from build123d import *

# Parameters (mm, degrees)
BOSS_EXTRUDE1_DEPTH = 1.5


with BuildPart() as part:
    # Sketch1 → Boss-Extrude1 (new body, symmetric)
    with BuildSketch(Plane(origin=(0, 0, 0), x_dir=(1, 0, 0), z_dir=(0, 1, 0))):
        with BuildLine():
            Line((-94.5, 0), (-88.5, 0))
            Line((-88.5, 0), (-88.5, 5))
            Line((-88.5, 5), (-84, 5))
            ThreePointArc((-84, 5), (0, 89), (84, 5))
            Line((84, 5), (88.5, 5))
            Line((88.5, 5), (88.5, 0))
            Line((88.5, 0), (94.5, 0))
            Line((94.5, 0), (94.5, 5))
            Line((94.5, 5), (99, 5))
            ThreePointArc((99, 5), (0, 104), (-99, 5))
            Line((-99, 5), (-94.5, 5))
            Line((-94.5, 5), (-94.5, 0))
        make_face()
    extrude(amount=BOSS_EXTRUDE1_DEPTH, both=True)


solid = part.part
Could you check a few things on this model? Use its own coordinates, in mm. Round coordinates to 2 decimals unless told otherwise and drop trailing zeros. Order: outer loops, then holes, each group sorted by start corner. A loop starts at its lowest first (then second) coordinate and runs counter-clockwise, first axis right, second up.
Q1. Imagine slicing it at D-D, the plane x = -59. List the corners of the cut face in (y, z) for me.
Geometry says:
outline: (-1.5, -84.5) - (1.5, -84.5) - (1.5, -64.79) - (-1.5, -64.79) - close
Q2. Please list where these lines run through material, in increasing order: probe 1 along X at (y, z) = (1.1, -21); probe 2 along X at (y, z) = (-0.2, -36); probe 3 along Z at (x, y) = (72, 0.8).
Geometry says:
probe 1: x = -97.7 to -82.46, 82.46 to 97.7
probe 2: x = -94.02 to -78.07, 78.07 to 94.02
probe 3: z = -72.95 to -48.27
Q3. Imagine slicing it at B-B, the plane y = -0.9. List the corners of the cut face in (x, z) for me.
Geometry says:
outline: (-99, -5) arc R99 ccw to (99, -5) - (94.5, -5) - (94.5, 0) - (88.5, 0) - (88.5, -5) - (84, -5) arc R84 cw to (-84, -5) - (-88.5, -5) - (-88.5, 0) - (-94.5, 0) - (-94.5, -5) - close
Q4. Imagine slicing it at A-A, the plane z = -86.5. List the corners of the cut face in (x, y) for me, then the cut area to 3 significant figures.
Geometry says:
outline: (-56.2, -1.5) - (-20.34, -1.5) - (-20.34, 1.5) - (-56.2, 1.5) - close; (20.34, -1.5) - (56.2, -1.5) - (56.2, 1.5) - (20.34, 1.5) - close
area: 215 mm2
Q5. Thinking about a two-plate mould opening in X: for faces 1 (the face through (2.177, 0.021, -103.976)), 2 (the face through (0, 1.5, -91)), 3 (the face through (-1.85, 0.02, -88.98)), which applies, released by +X, released by -X, zero draft, split by the parting line, or undercut?
Geometry says:
face 1: split by the parting line
face 2: zero draft
face 3: undercut
Q6. I'm going to push flat-ended pins straight in: P1, Ø1, axis at y = -0.5, z = -60.5, coming from the -X side; P2, Ø1.5, axis at x = 23, y = 1, coming from the +Z side; P3, Ø1.5, axis at y = -0.5, z = -2, coming from the +X side. Where does each tip first touch, or does it pass through?
Geometry says:
P1: stops at x = -82.32
P2: stops at z = -85.57
P3: stops at x = 94.5
Q7. Imagine slicing it at C-C, the plane z = -41. List the corners of the cut face in (x, y) for me.
Geometry says:
outline: (-92.22, -1.5) - (-75.89, -1.5) - (-75.89, 1.5) - (-92.22, 1.5) - close; (75.89, -1.5) - (92.22, -1.5) - (92.22, 1.5) - (75.89, 1.5) - close
